from build123d import *

# Parameters (mm, degrees)
SKETCH1_W           = 63.27
SKETCH1_H           = 63.27
BOSS_EXTRUDE1_DEPTH = 2
SKETCH2_R           = 6
CUT_EXTRUDE1_DEPTH  = 2
SKETCH3_W           = 16
SKETCH3_H           = 62
BOSS_EXTRUDE2_DEPTH = 2
SKETCH4_W           = 16
SKETCH4_H           = 63.27
CUT_EXTRUDE2_DEPTH  = 10
SKETCH5_W           = 47.27
SKETCH5_H           = 16
CUT_EXTRUDE3_DEPTH  = 10
SKETCH6_W           = 31.27
SKETCH6_H           = 16
CUT_EXTRUDE4_DEPTH  = 10


with BuildPart() as part:
    # Sketch1 → Boss-Extrude1 (new body)
    with BuildSketch(Plane(origin=(0, 0, 0), x_dir=(1, 0, 0), z_dir=(0, 1, 0))):
        Rectangle(SKETCH1_W, SKETCH1_H)
    extrude(amount=BOSS_EXTRUDE1_DEPTH)

    # Sketch2 → Cut-Extrude1 (cut)
    with BuildSketch(Plane(origin=(0, 2, 0), x_dir=(1, 0, 0), z_dir=(0, 1, 0))):
        with Locations(Location((0, 0, 0), (0, 0, 270))):
            Circle(SKETCH2_R)
    extrude(amount=-CUT_EXTRUDE1_DEPTH, mode=Mode.SUBTRACT)

    # Sketch3 → Boss-Extrude2 (add)
    with BuildSketch(Plane(origin=(0, 2, 0), x_dir=(1, 0, 0), z_dir=(0, 1, 0))):
        with Locations((23.635, 31)):
            Rectangle(SKETCH3_W, SKETCH3_H)
    extrude(amount=-BOSS_EXTRUDE2_DEPTH)

    # Sketch4 → Cut-Extrude2 (cut)
    with BuildSketch(Plane.XZ):
        with Locations((-23.635, 0)):
            Rectangle(SKETCH4_W, SKETCH4_H)
    extrude(amount=-CUT_EXTRUDE2_DEPTH, mode=Mode.SUBTRACT)

    # Sketch5 → Cut-Extrude3 (cut)
    with BuildSketch(Plane.XZ):
        with Locations((8, 23.635)):
            Rectangle(SKETCH5_W, SKETCH5_H)
    extrude(amount=-CUT_EXTRUDE3_DEPTH, mode=Mode.SUBTRACT)

    # Sketch6 → Cut-Extrude4 (cut)
    with BuildSketch(Plane.XZ):
        with Locations((0, -23.635)):
            Rectangle(SKETCH6_W, SKETCH6_H)
    extrude(amount=-CUT_EXTRUDE4_DEPTH, mode=Mode.SUBTRACT)


solid = part.part
The model under review builds one solid part; all positions refer to its coordinate system, in mm. A direction names the side the tool comes from. Round coordinates to 2 decimals unless told otherwise and drop trailing zeros. Loops run counter-clockwise (first coordinate to the right, second up) from the corner with the lowest first, then second, coordinate; pieces in that order, holes last. Notation, with made-up numbers: (79.5, 81.25) - (125.5, 81.25) arc R23 cw to (125.5, 89.25) - close; hole circle Ø9 at (12.25, 56.25). An arc over 180 degrees is marked (long way). Use CSV: the item, a comma, the result in double quotes.
(1) The part is to be moulded in two halves that separate along Z. For faces 1 (the flat face through (8, 1, 15.635)), 2 (the cylindrical face through (1.802, 1.014, 5.723)), 3 (the flat face through (-15.635, 1, 0)), say which applies: pulls with the +Z half, pulls with the -Z half, needs draft (parallel to the pull), parting line crosses it, or undercut.
Working result:
face 1,"pulls with the +Z half"
face 2,"undercut"
face 3,"needs draft"
(2) Machinability: for faces 4 (the flat face through (24, 1, -62)), 5 (the flat face through (0, 1, -15.635)), which of the approach directions +Z, -Z, +X, -X, +Y, -Y give a long, thin tool a straight path to every point of the face, cutting with its end or side? Answer none if there is none.
Working result:
face 4,"-Z, +X, -X, +Y, -Y"
face 5,"-Z, -X, +Y, -Y"
(3) Take a section at D-D, the plane x = 13.5. Give the boundary of the cut face in (y, z) (3 decimals), plus the area to 3 significant figures.
Working result:
outline,"(0, -15.635) - (2, -15.635) - (2, 15.635) - (0, 15.635) - close"
area,"62.5 mm^2"
(4) Take a section at C-C, the plane y = 1.7. Give the boundary of the cut face in (x, z) (3 decimals).
Working result:
outline,"(-15.635, -15.635) - (15.635, -15.635) - (15.635, -62) - (31.635, -62) - (31.635, 15.635) - (-15.635, 15.635) - close; hole circle Ø12 at (0, 0)"
(5) Take a section at A-A, the plane x = 0. Give the boundary of the cut face in (y, z) (3 decimals).
Working result:
outline,"(0, -15.635) - (2, -15.635) - (2, -6) - (0, -6) - close; (0, 6) - (2, 6) - (2, 15.635) - (0, 15.635) - close"
(6) Clearance check with flat-ended pins moving along their axes: P1, Ø1, axis at y = 1, z = -42, coming from the -X side (3 decimals); P2, Ø1, axis at x = 8.5, y = 1, coming from the -Z side (3 decimals). State where each tip first meets the part, or that it passes through.
Working result:
P1,"stops at x = 15.635"
P2,"stops at z = -15.635"
(7) Take a section at B-B, the plane z = 0. Give the boundary of the cut face in (x, y) (3 decimals), plus the area to 3 significant figures.
Working result:
outline,"(-15.635, 0) - (-6, 0) - (-6, 2) - (-15.635, 2) - close; (6, 0) - (31.635, 0) - (31.635, 2) - (6, 2) - close"
area,"70.5 mm^2"
(8) For line 1 (X direction, y = 1.15, z = 0) (3 decimals); line 2 (X direction, y = 0.8, z = -42) (3 decimals); line 3 (Z direction, x = -12, y = 1.75) (3 decimals), list the stretches that pass through material, from the lowest coordinate up.
Working result:
line 1,"x = -15.635 to -6, 6 to 31.635"
line 2,"x = 15.635 to 31.635"
line 3,"z = -15.635 to 15.635"
